Part model, mm, in its own coordinate system. A direction names the side the tool comes from. Give positions to 0.01 mm unless a question says otherwise; leave off trailing zeros. Write each loop counter-clockwise with the first axis right and the second up, starting at its lowest first coordinate (ties: lowest second). Pieces come first, ordered by that corner, then holes.
from build123d import *

# Parameters (mm, degrees)
SKETCH2_W               = 70
SKETCH2_H               = 70
BOSS_EXTRUDE1_DEPTH     = 24
SKETCH3_R               = 55
SKETCH3_W               = 70
SKETCH3_H               = 70
SKETCH3_R_2             = 22
SKETCH3_R_3             = 16
CUT_EXTRUDE1_DEPTH      = 4
SKETCH3_3_W             = 70
SKETCH3_3_H             = 70
SKETCH3_3_R             = 25
CUT_EXTRUDE2_DEPTH      = 4
SKETCH4_W               = 20
SKETCH4_H               = 20
SKETCH4_R               = 4.25
CUT_EXTRUDE3_DEPTH      = 10
CUT_EXTRUDE4_REACH      = 57.009
SKETCH4_3_R             = 4.25
MIRROR2_COPY_1_SKETCH_W = 20
MIRROR2_COPY_1_SKETCH_H = 20
MIRROR2_COPY_1_SKETCH_R = 4.25
MIRROR2_COPY_1_DEPTH    = 10
MIRROR2_COPY_2_REACH    = 57.009
MIRROR2_COPY_2_SKETCH_R = 4.25
FILLET1_R               = 10
SKETCH5_R               = 17.5
BOSS_EXTRUDE2_DEPTH     = 20
SKETCH6_R               = 14
CUT_EXTRUDE5_DEPTH      = 8
SKETCH7_R               = 9
CUT_EXTRUDE6_DEPTH      = 2
SKETCH8_R               = 10
CUT_EXTRUDE7_DEPTH      = 10
SKETCH9_R               = 9
CUT_EXTRUDE8_DEPTH      = 4
SKETCH10_R              = 10
CUT_EXTRUDE9_DEPTH      = 20
SKETCH11_R              = 7.5
CUT_EXTRUDE10_DEPTH     = 1
M10_TAPPED_HOLE1_REACH  = 91.006
M10_TAPPED_HOLE1_BORE_R = 4.25
CHAMFER1_SIZE           = 1


with BuildPart() as part:
    # Sketch2 → Boss-Extrude1 (new body)
    with BuildSketch(Plane.XY):
        Rectangle(SKETCH2_W, SKETCH2_H)
    extrude(amount=BOSS_EXTRUDE1_DEPTH)

    # Sketch3 → Cut-Extrude1 (cut)
    # profile 1 of 2: a face of its own
    with BuildSketch(Plane(origin=(0, 0, 0), x_dir=(-1, 0, 0), z_dir=(0, 0, -1))):
        Circle(SKETCH3_R)
        Rectangle(SKETCH3_W, SKETCH3_H, mode=Mode.SUBTRACT)
    # profile 2 of 2: a face of its own
    with BuildSketch(Plane(origin=(0, 0, 0), x_dir=(-1, 0, 0), z_dir=(0, 0, -1))):
        Circle(SKETCH3_R_2)
        Circle(SKETCH3_R_3, mode=Mode.SUBTRACT)
    extrude(amount=-CUT_EXTRUDE1_DEPTH, mode=Mode.SUBTRACT)

    # Sketch3<3> → Cut-Extrude2 (cut)
    with BuildSketch(Plane(origin=(0, 0, 0), x_dir=(-1, 0, 0), z_dir=(0, 0, -1))):
        Rectangle(SKETCH3_3_W, SKETCH3_3_H)
        Circle(SKETCH3_3_R, mode=Mode.SUBTRACT)
    extrude(amount=-CUT_EXTRUDE2_DEPTH, mode=Mode.SUBTRACT)

    # Sketch4 → Cut-Extrude3 (cut)
    with BuildSketch(Plane.XY.offset(24)):
        with Locations((-25, 25)):
            Rectangle(SKETCH4_W, SKETCH4_H)
        with Locations((-25, 25)):
            Circle(SKETCH4_R, mode=Mode.SUBTRACT)
    cut_extrude3 = extrude(amount=-CUT_EXTRUDE3_DEPTH, mode=Mode.SUBTRACT)

    # Sketch4<3> → Cut-Extrude4 (cut, up to next)
    with BuildSketch(Plane.XY.offset(24), mode=Mode.PRIVATE) as cut_extrude4_sk1:
        with Locations((-25, 25)):
            Circle(SKETCH4_3_R)
    cut_extrude4_tool1 = extrude(cut_extrude4_sk1.sketch, amount=-CUT_EXTRUDE4_REACH, mode=Mode.PRIVATE) & part.part
    cut_extrude4 = cut_extrude4_tool1.solids().sort_by_distance((-25, 25, 24))[0]
    add(cut_extrude4, mode=Mode.SUBTRACT)

    # Mirror1: Cut-Extrude3, Cut-Extrude4 across plane
    add(cut_extrude3.mirror(Plane.ZX), mode=Mode.SUBTRACT)
    add(cut_extrude4.mirror(Plane.ZX), mode=Mode.SUBTRACT)

    # Mirror2: Cut-Extrude3, Cut-Extrude4 across plane
    add(cut_extrude3.mirror(Plane(origin=(0, 0, 0), x_dir=(0, 0, 1), z_dir=(1, 0, 0))), mode=Mode.SUBTRACT)
    add(cut_extrude4.mirror(Plane(origin=(0, 0, 0), x_dir=(0, 0, 1), z_dir=(1, 0, 0))), mode=Mode.SUBTRACT)

    # Mirror2 copy 1 sketch → Mirror2 copy 1 (cut)
    with BuildSketch(Plane(origin=(0, 0, 24), x_dir=(-1, 0, 0), z_dir=(0, 0, 1))):
        with Locations((-25, 25)):
            Rectangle(MIRROR2_COPY_1_SKETCH_W, MIRROR2_COPY_1_SKETCH_H)
        with Locations((-25, 25)):
            Circle(MIRROR2_COPY_1_SKETCH_R, mode=Mode.SUBTRACT)
    extrude(amount=-MIRROR2_COPY_1_DEPTH, mode=Mode.SUBTRACT)

    # Mirror2 copy 2 sketch → Mirror2 copy 2 (cut, up to next)
    with BuildSketch(Plane(origin=(0, 0, 24), x_dir=(-1, 0, 0), z_dir=(0, 0, 1)), mode=Mode.PRIVATE) as mirror2_copy_2_sk1:
        with Locations((-25, 25)):
            Circle(MIRROR2_COPY_2_SKETCH_R)
    mirror2_copy_2_tool1 = extrude(mirror2_copy_2_sk1.sketch, amount=-MIRROR2_COPY_2_REACH, mode=Mode.PRIVATE) & part.part
    add(mirror2_copy_2_tool1.solids().sort_by_distance((25, -25, 24))[0], mode=Mode.SUBTRACT)

    # Fillet1
    fillet1_edges = [part.edges().sort_by_distance(p)[0] for p in [
        (35, -35, 9),
        (15, -15, 19),
        (-35, 35, 9),
        (-15, 15, 19),
        (-35, -35, 9),
        (-15, -15, 19),
        (35, 35, 9),
        (15, 15, 19),
    ]]
    fillet(fillet1_edges, radius=FILLET1_R)

    # Sketch5 → Boss-Extrude2 (add)
    with BuildSketch(Plane.XY.offset(24)):
        Circle(SKETCH5_R)
    extrude(amount=BOSS_EXTRUDE2_DEPTH)

    # Sketch6 → Cut-Extrude5 (cut)
    with BuildSketch(Plane.XY.offset(44)):
        Circle(SKETCH6_R)
    extrude(amount=-CUT_EXTRUDE5_DEPTH, mode=Mode.SUBTRACT)

    # Sketch7 → Cut-Extrude6 (cut)
    with BuildSketch(Plane.XY.offset(36)):
        Circle(SKETCH7_R)
    extrude(amount=-CUT_EXTRUDE6_DEPTH, mode=Mode.SUBTRACT)

    # Sketch8 → Cut-Extrude7 (cut)
    with BuildSketch(Plane.XY.offset(34)):
        Circle(SKETCH8_R)
    extrude(amount=-CUT_EXTRUDE7_DEPTH, mode=Mode.SUBTRACT)

    # Sketch9 → Cut-Extrude8 (cut)
    with BuildSketch(Plane.XY.offset(24)):
        Circle(SKETCH9_R)
    extrude(amount=-CUT_EXTRUDE8_DEPTH, mode=Mode.SUBTRACT)

    # Sketch10 → Cut-Extrude9 (cut)
    with BuildSketch(Plane.XY.offset(20)):
        Circle(SKETCH10_R)
    extrude(amount=-CUT_EXTRUDE9_DEPTH, mode=Mode.SUBTRACT)

    # Sketch11 → Cut-Extrude10 (cut)
    with BuildSketch(Plane(origin=(35, 0, 0), x_dir=(0, 0, -1), z_dir=(1, 0, 0))):
        with Locations((-14, 0)):
            Circle(SKETCH11_R)
    extrude(amount=-CUT_EXTRUDE10_DEPTH, mode=Mode.SUBTRACT)

    # M10 Tapped Hole1 bore → M10 Tapped Hole1 (cut, up to next)
    with BuildSketch(Plane(origin=(34, 0, 0), x_dir=(0, 0, -1), z_dir=(1, 0, 0)), mode=Mode.PRIVATE) as m10_tapped_hole1_sk1:
        with Locations((-14, 0)):
            Circle(M10_TAPPED_HOLE1_BORE_R)
    m10_tapped_hole1_tool1 = extrude(m10_tapped_hole1_sk1.sketch, amount=-M10_TAPPED_HOLE1_REACH, mode=Mode.PRIVATE) & part.part
    add(m10_tapped_hole1_tool1.solids().sort_by_distance((34, 0, 14))[0], mode=Mode.SUBTRACT)

    # Chamfer1
    chamfer1_edges = [part.edges().sort_by_distance(p)[0] for p in [
        (34, 0, 18.25),
    ]]
    chamfer(chamfer1_edges, length=CHAMFER1_SIZE)


solid = part.part
1) Saw through at A-A (z = 22.5). Write the cut outline in (x, y), and give its area (3 significant figures).
Check result:
outline: (-35, -15) - (-25, -15) arc R10 cw to (-15, -25) - (-15, -35) - (15, -35) - (15, -25) arc R10 cw to (25, -15) - (35, -15) - (35, 15) - (25, 15) arc R10 cw to (15, 25) - (15, 35) - (-15, 35) - (-15, 25) arc R10 cw to (-25, 15) - (-35, 15) - close; hole circle Ø18 at (0, 0)
area: 3,130 mm2
2) Mould opens along Y. For faces 6 (the flat face through (30, -15, 19)), 7 (the flat face through (15, 30, 19)), 8 (the cylindrical face through (21.194, 1.277, 9.946)) say: +Y half, -Y half, draft (parallel to the pull), parting line (faces both ways), or undercut.
Check result:
face 6: -Y half
face 7: draft
face 8: undercut
3) Saw through at B-B (x = -24). Write the cut outline in (y, z), and give its area (3 significant figures).
Check result:
outline: (-35, 4) - (-29.13, 4) - (-29.13, 14) - (-35, 14) - close; (-20.87, 4) - (-7, 4) - (-7, 0) - (7, 0) - (7, 4) - (20.87, 4) - (20.87, 14) - (15.05, 14) - (15.05, 24) - (-15.05, 24) - (-15.05, 14) - (-20.87, 14) - close; (29.13, 4) - (35, 4) - (35, 14) - (29.13, 14) - close
area: 892 mm2
4) Flat gauge pins, fed straight in: P1, Ø5, axis at x = 31, z = 21, coming from the +Y side; P2, Ø5, axis at x = 20, y = 13, coming from the +Z side; P3, Ø13.5, axis at x = 25, y = 25, coming from the -Z side. Where does each tip first touch, or does it go through?
Check result:
P1: stops at y = 15
P2: stops at z = 24
P3: stops at z = 4
5) 3-axis set-ups, long thin cutter, end or side, ignore diameter. For faces 1 (the flat face through (-30, -15, 19)), 2 (the flat face through (24, 8, 4)), 3 (the flat face through (-30, 25, 14)), 4 (the flat face through (30, 25, 14)), 5 (the flat face through (15, -30, 19)): which of +Z, -Z, +X, -X, +Y, -Y reach the whole face in a straight line?
Check result:
face 1: +Z, -X, -Y
face 2: -Z
face 3: +Z, -X, +Y
face 4: +Z, +X, +Y
face 5: +Z, +X, -Y
6) Saw through at C-C (y = -2). State how many separate pieces and enclosed holes the cut face has, and give its area (3 significant figures).
Check result:
separate pieces: 3
enclosed holes: 0
area: 1,130 mm2
7) Drill centre lines: L1, parallel to Y at x = 25, z = 6; L2, parallel to X at y = 28, z = 5.5. Where is each one in solid material? Low to high.
Check result:
L1: y = -35 to -29.25, -20.75 to 20.75, 29.25 to 35
L2: x = -34.54 to -28.01, -21.99 to 21.99, 28.01 to 34.54
8) Saw through at D-D (z = 40.5). Write the cut outline in (x, y).
Check result:
outline: circle Ø35 at (0, 0); hole circle Ø28 at (0, 0)
